Geometry: final body of the model. Coordinates: model frame, mm. Round coordinates to 2 decimals unless told otherwise and drop trailing zeros. Order: outer loops, then holes, each group sorted by start corner. A loop starts at its lowest first (then second) coordinate and runs counter-clockwise, first axis right, second up. Notation, with made-up numbers: M -1.75,64.25 L 35.25,64.25 A20 ccw 35.25,95.25 Z; hole C 16.5,38.25 d8. An arc over 180 degrees is marked long. Put each result on its own line as item: value. Start each with the question number.
1) Section A-A, the plane x = 8. Return loops of the section in (y, z).
2) First-contact query: P1, Ø3, axis at x = 47, y = -67.5, coming from the -Z side; P2, Ø1.5, axis at x = 46, z = 3, coming from the +Y side. Flat tips, straight axial feed; report the tip coordinate or a pass-through.
3) Section C-C, the plane z = 2.5. Count the separate pieces of the cut face and the enclosed holes in it, then the cut area to 3 significant figures.
4) Material intervals for probe 1 along X at (y, z) = (-3.5, 0.3); probe 2 along Y at (x, z) = (22.5, 0.6); probe 3 along Y at (x, z) = (49.5, 0.95), sorted ascending. Write a range as [from, to].
5) Section B-B, the plane y = -32. Return loops of the section in (x, z).
from build123d import *

# Parameters (mm, degrees)
F0_W         = 67
F0_H         = 77
F1_DEPTH     = 3.5
F2_R         = 5
F3_T1_DEPTH  = 57
F3_T3_DEPTH  = 67
F3_T6_ANGLE  = 90
F3_T8_ANGLE  = 90
F3_T10_ANGLE = 90
F3_T12_ANGLE = 90
F5_DEPTH     = 3.5


# Not quite as in the source:
# - a fillet or chamfer that OpenCascade refuses, or shapes differently, is made with other operations: its cross-section is extruded or revolved along the edge and cut away or added


with BuildPart() as f1:
    # F0 (on Top) → F1 (new body)
    with BuildSketch(Plane.XY):
        with Locations((33.5, -38.5)):
            Rectangle(F0_W, F0_H)
    extrude(amount=F1_DEPTH)

    # F2
    f2_edges = [f1.edges().sort_by_distance(p)[0] for p in [
        (67, -77, 1.75),
        (67, 0, 1.75),
        (0, 0, 1.75),
        (0, -77, 1.75),
    ]]
    fillet(f2_edges, radius=F2_R)

    # F3: fillet of radius 5 on 8 edges, made by hand

    # F3_s2 → F3_t1 (cut)
    with BuildSketch(Plane.YZ.offset(5)):
        with BuildLine():
            ThreePointArc((0, 0), (-1.8116561155, 2.5311288741), (-4.7696960071, 3.5))
            Line((-4.7696960071, 3.5), (0, 3.5))
            Line((0, 3.5), (0, 0))
        make_face()
        with BuildLine():
            ThreePointArc((-72.2303039929, 3.5), (-75.1883438845, 2.5311288741), (-77, 0))
            Line((-77, 0), (-77, 3.5))
            Line((-77, 3.5), (-72.2303039929, 3.5))
        make_face()
    extrude(amount=F3_T1_DEPTH, mode=Mode.SUBTRACT)

    # F3_s4 → F3_t3 (cut)
    with BuildSketch(Plane.XZ.offset(5)):
        with BuildLine():
            ThreePointArc((62.2303039929, 3.5), (65.1883438845, 2.5311288741), (67, 0))
            Line((67, 0), (67, 3.5))
            Line((67, 3.5), (62.2303039929, 3.5))
        make_face()
        with BuildLine():
            ThreePointArc((4.7696960071, 3.5), (1.8116561155, 2.5311288741), (0, 0))
            Line((0, 0), (0, 3.5))
            Line((0, 3.5), (4.7696960071, 3.5))
        make_face()
    extrude(amount=F3_T3_DEPTH, mode=Mode.SUBTRACT)

    # F3_s5 → F3_t6 (revolve, cut)
    with BuildSketch(Plane.YZ.offset(62)):
        with BuildLine():
            ThreePointArc((0, 0), (-1.8116561155, 2.5311288741), (-4.7696960071, 3.5))
            Line((-4.7696960071, 3.5), (0, 3.5))
            Line((0, 3.5), (0, 0))
        make_face()
    revolve(axis=Axis((62, -5, 3.5), (0, 0, -1)), revolution_arc=F3_T6_ANGLE, mode=Mode.SUBTRACT)

    # F3_s7 → F3_t8 (revolve, cut)
    with BuildSketch(Plane.YZ.offset(5)):
        with BuildLine():
            ThreePointArc((0, 0), (-1.8116561155, 2.5311288741), (-4.7696960071, 3.5))
            Line((-4.7696960071, 3.5), (0, 3.5))
            Line((0, 3.5), (0, 0))
        make_face()
    revolve(axis=Axis((5, -5, 3.5), (0, 0, 1)), revolution_arc=F3_T8_ANGLE, mode=Mode.SUBTRACT)

    # F3_s9 → F3_t10 (revolve, cut)
    with BuildSketch(Plane.YZ.offset(62)):
        with BuildLine():
            ThreePointArc((-72.2303039929, 3.5), (-75.1883438845, 2.5311288741), (-77, 0))
            Line((-77, 0), (-77, 3.5))
            Line((-77, 3.5), (-72.2303039929, 3.5))
        make_face()
    revolve(axis=Axis((62, -72, 3.5), (0, 0, 1)), revolution_arc=F3_T10_ANGLE, mode=Mode.SUBTRACT)

    # F3_s11 → F3_t12 (revolve, cut)
    with BuildSketch(Plane.XZ.offset(72)):
        with BuildLine():
            ThreePointArc((4.7696960071, 3.5), (1.8116561155, 2.5311288741), (0, 0))
            Line((0, 0), (0, 3.5))
            Line((0, 3.5), (4.7696960071, 3.5))
        make_face()
    revolve(axis=Axis((5, -72, 3.5), (0, 0, 1)), revolution_arc=F3_T12_ANGLE, mode=Mode.SUBTRACT)

    # F4 (on face) → F5 (cut)
    with BuildSketch(Plane.XY.offset(3.5)):
        with BuildLine():
            Line((62.2303039929, -72), (63.7, -72))
            ThreePointArc((63.7, -72), (63.5705952053, -71.349438165), (63.202081528, -70.797918472))
            Line((63.202081528, -70.797918472), (62.2303039929, -71.7696960071))
            Line((62.2303039929, -71.7696960071), (62.2303039929, -72))
        make_face()
        with BuildLine():
            ThreePointArc((63.202081528, -70.797918472), (62.7556933452, -70.4771974626), (62.2303039929, -70.3156722199))
            Line((62.2303039929, -70.3156722199), (62.2303039929, -71.7696960071))
            Line((62.2303039929, -71.7696960071), (63.202081528, -70.797918472))
        make_face()
        with BuildLine():
            ThreePointArc((62.2303039929, -70.3156722199), (60.8823052268, -70.7190790836), (60.3, -72))
            Line((60.3, -72), (62, -72))
            Line((62, -72), (62.2303039929, -71.7696960071))
            Line((62.2303039929, -71.7696960071), (62.2303039929, -70.3156722199))
        make_face()
        with BuildLine():
            Line((62, -72.2303039929), (60.3156722199, -72.2303039929))
            ThreePointArc((60.3156722199, -72.2303039929), (62.1154183127, -73.6960774195), (63.7, -72))
            Line((63.7, -72), (62.2303039929, -72))
            ThreePointArc((62.2303039929, -72), (62.1628495151, -72.1628495151), (62, -72.2303039929))
        make_face()
        with BuildLine():
            ThreePointArc((60.3, -72), (60.3039225805, -72.1154183127), (60.3156722199, -72.2303039929))
            Line((60.3156722199, -72.2303039929), (62, -72.2303039929))
            ThreePointArc((62, -72.2303039929), (62.1628495151, -72.1628495151), (62.2303039929, -72))
            Line((62.2303039929, -72), (62, -72))
            Line((62, -72), (60.3, -72))
        make_face()
        Polygon((62.2303039929, -71.7696960071), (62, -72), (62.2303039929, -72), align=None)
        with BuildLine():
            Line((4.7696960071, -72), (3.3, -72))
            ThreePointArc((3.3, -72), (4.8845816873, -73.6960774195), (6.6843277801, -72.2303039929))
            Line((6.6843277801, -72.2303039929), (5, -72.2303039929))
            ThreePointArc((5, -72.2303039929), (4.8371504849, -72.1628495151), (4.7696960071, -72))
        make_face()
        with BuildLine():
            ThreePointArc((4.7696960071, -70.3156722199), (3.7190790836, -70.8823052268), (3.3, -72))
            Line((3.3, -72), (4.7696960071, -72))
            Line((4.7696960071, -72), (4.7696960071, -70.3156722199))
        make_face()
        with BuildLine():
            Line((4.7696960071, -70.3156722199), (4.7696960071, -72))
            Line((4.7696960071, -72), (6.7, -72))
            ThreePointArc((6.7, -72), (6.1176947732, -70.7190790836), (4.7696960071, -70.3156722199))
        make_face()
        with BuildLine():
            Line((6.7, -72), (4.7696960071, -72))
            ThreePointArc((4.7696960071, -72), (4.8371504849, -72.1628495151), (5, -72.2303039929))
            Line((5, -72.2303039929), (6.6843277801, -72.2303039929))
            ThreePointArc((6.6843277801, -72.2303039929), (6.6960774195, -72.1154183127), (6.7, -72))
        make_face()
        with BuildLine():
            Line((5, -4.7696960071), (5, -3.3))
            ThreePointArc((5, -3.3), (3.797918472, -3.797918472), (3.3, -5))
            Line((3.3, -5), (4.7696960071, -5))
            ThreePointArc((4.7696960071, -5), (4.8371504849, -4.8371504849), (5, -4.7696960071))
        make_face()
        with BuildLine():
            ThreePointArc((6.6843277801, -4.7696960071), (6.1176947732, -3.7190790836), (5, -3.3))
            Line((5, -3.3), (5, -4.7696960071))
            Line((5, -4.7696960071), (6.6843277801, -4.7696960071))
        make_face()
        with BuildLine():
            Line((6.6843277801, -4.7696960071), (5, -4.7696960071))
            Line((5, -4.7696960071), (5, -5))
            Line((5, -5), (4.7696960071, -5))
            Line((4.7696960071, -5), (4.7696960071, -6.6843277801))
            ThreePointArc((4.7696960071, -6.6843277801), (6.1176947732, -6.2809209164), (6.7, -5))
            ThreePointArc((6.7, -5), (6.6960774195, -4.8845816873), (6.6843277801, -4.7696960071))
        make_face()
        with BuildLine():
            Line((4.7696960071, -5), (3.3, -5))
            ThreePointArc((3.3, -5), (3.7190790836, -6.1176947732), (4.7696960071, -6.6843277801))
            Line((4.7696960071, -6.6843277801), (4.7696960071, -5))
        make_face()
        with BuildLine():
            Line((5, -5), (5, -4.7696960071))
            ThreePointArc((5, -4.7696960071), (4.8371504849, -4.8371504849), (4.7696960071, -5))
            Line((4.7696960071, -5), (5, -5))
        make_face()
        with BuildLine():
            Line((62, -4.7696960071), (60.3156722199, -4.7696960071))
            ThreePointArc((60.3156722199, -4.7696960071), (60.797918472, -6.202081528), (62.2303039929, -6.6843277801))
            Line((62.2303039929, -6.6843277801), (62.2303039929, -5))
            ThreePointArc((62.2303039929, -5), (62.1628495151, -4.8371504849), (62, -4.7696960071))
        make_face()
        with BuildLine():
            ThreePointArc((63.7, -5), (62.1154183127, -3.3039225805), (60.3156722199, -4.7696960071))
            Line((60.3156722199, -4.7696960071), (62, -4.7696960071))
            ThreePointArc((62, -4.7696960071), (62.1628495151, -4.8371504849), (62.2303039929, -5))
            Line((62.2303039929, -5), (62.2303039929, -6.6843277801))
            ThreePointArc((62.2303039929, -6.6843277801), (63.2809209164, -6.1176947732), (63.7, -5))
        make_face()
    extrude(amount=-F5_DEPTH, mode=Mode.SUBTRACT)


solid = f1.part
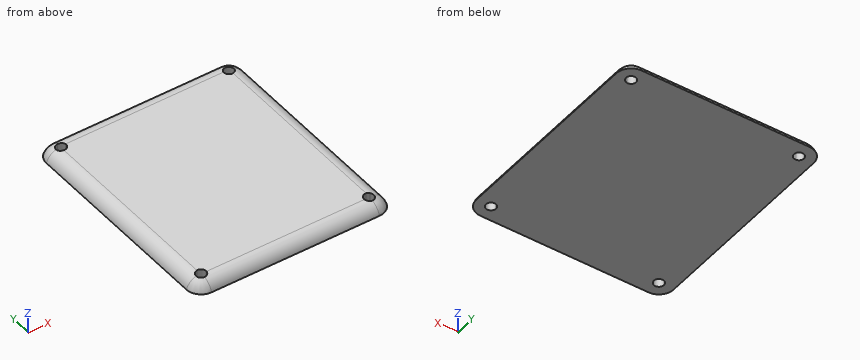
Result sheet:
1. outline: M -77,0 L 0,0 A5 ccw -4.77,3.5 L -72.23,3.5 A5 ccw Z
2. P1: stops at z = 0
2. P2: stops at y = -1.46
3. separate pieces: 1
3. enclosed holes: 4
3. area: 4,620 mm2
4. probe 1: x = [0.34, 4.2], [5.8, 61.2], [62.8, 66.66]
4. probe 2: y = [-76.77, -0.23]
4. probe 3: y = [-76.59, -0.41]
5. outline: M 0,0 L 67,0 A5 ccw 62.23,3.5 L 4.77,3.5 A5 ccw Z
